Geometry: final body of the model. Coordinates: model frame, mm. Face numbers are marked on the shaded views. A direction names the side the tool comes from. Round coordinates to 2 decimals unless told otherwise and drop trailing zeros. Write each loop counter-clockwise with the first axis right and the second up, starting at its lowest first coordinate (ties: lowest second). Pieces come first, ordered by that corner, then holes. Notation, with made-up numbers: (40.5, 86.5) -> (75.5, 86.5) arc R15 cw to (75.5, 104.5) -> close; hole circle Ø3 at (80.5, -16.5). An arc over 180 degrees is marked (long way). One line per item, written item: value. Start each with the question number.
from build123d import *

# Parameters (mm, degrees)
CROQUIS3_R                 = 12
SALIENTE_EXTRUIR1_DEPTH    = 4
CROQUIS4_R                 = 3.95
SALIENTE_EXTRUIR2_DEPTH    = 35
CORTAR_EXTRUIR1_START      = -20
CORTAR_EXTRUIR1_DEPTH      = 20
CROQUIS7_R                 = 12
CORTAR_EXTRUIR2_DEPTH      = 2
CORTAR_EXTRUIR3_DEPTH      = 41.706264874
CORTAR_EXTRUIR3_DEPTH_BACK = 41.706264874
CROQUIS8_R                 = 0.726366889


with BuildPart() as part:
    # Croquis3 → Saliente-Extruir1 (new body)
    with BuildSketch(Plane(origin=(0, 0, 0), x_dir=(1, 0, 0), z_dir=(0, 1, 0))):
        with Locations(Location((0, 0, 0), (0, 0, 270))):
            Circle(CROQUIS3_R)
    extrude(amount=SALIENTE_EXTRUIR1_DEPTH)

    # Croquis4 → Saliente-Extruir2 (add)
    with BuildSketch(Plane(origin=(0, 4, 0), x_dir=(1, 0, 0), z_dir=(0, 1, 0))):
        with Locations(Location((0, 0, 0), (0, 0, 270))):
            Circle(CROQUIS4_R)
    extrude(amount=SALIENTE_EXTRUIR2_DEPTH)

    # Croquis5 → Cortar-Extruir1 (cut)
    with BuildSketch(Plane(origin=(0, 39, 0), x_dir=(1, 0, 0), z_dir=(0, 1, 0)).offset(CORTAR_EXTRUIR1_START)):
        with BuildLine():
            Line((2.626785107, 2.95), (-2.626785107, 2.95))
            ThreePointArc((-2.626785107, 2.95), (0, 3.95), (2.626785107, 2.95))
        make_face()
    extrude(amount=CORTAR_EXTRUIR1_DEPTH, mode=Mode.SUBTRACT)

    # Croquis7 → Cortar-Extruir2 (cut)
    with BuildSketch(Plane.XZ):
        with Locations(Location((0, 0, 0), (0, 0, 270))):
            Circle(CROQUIS7_R)
    extrude(amount=-CORTAR_EXTRUIR2_DEPTH, mode=Mode.SUBTRACT)

    # Croquis8 → Cortar-Extruir3 (cut, two sides: drawn at the far end of the back side and taken through both)
    with BuildSketch(Plane.XZ.offset(-2).offset(-CORTAR_EXTRUIR3_DEPTH_BACK)):
        with Locations(Location((0, 8, 0), (0, 0, 270))):
            Circle(CROQUIS8_R)
        with Locations(Location((0, -8, 0), (0, 0, 270))):
            Circle(CROQUIS8_R)
    extrude(amount=CORTAR_EXTRUIR3_DEPTH + CORTAR_EXTRUIR3_DEPTH_BACK, mode=Mode.SUBTRACT)


solid = part.part
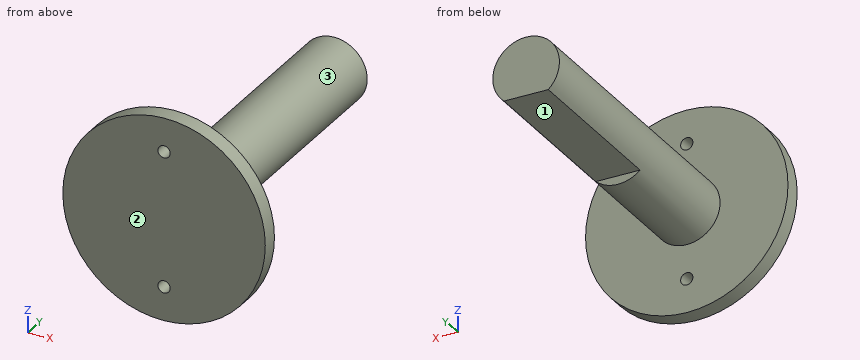
(1) Section query D-D (y = 21.5). Output: boundary loops of the cut face in (x, z), and give its area (3 significant figures).
(2) Pin query (flat end, axial travel): pin 1 (3 mm diameter, centred on x = -2.5, y = 26.5, fed in from -Z); pin 2 (12 mm diameter, centred on x = 6, z = 0.5, fed in from +Y); pin 3 (1 mm diameter, centred on x = 4, y = 15.5, fed in from +Z); pin 4 (12 mm diameter, centred on x = 0.5, y = 27.5, fed in from +Z). Return the tip coordinate at first contact, or that it passes through.
(3) Section query A-A (x = 0). Output: boundary loops of the cut face in (y, z).
(4) Set-up query: the marked faces 1, 2 and 3. Return all of +Z, -Z, +X, -X, +Y, -Y with unobstructed straight access to the full face (end or side cutting, diameter ignored); none if empty.
(5) Section query B-B (z = 8). Output: boundary loops of the cut face in (x, y), and give its area (3 significant figures).
(6) Line query: probe 1 along Y at (x, z) = (-6.5, -4); probe 2 along X at (y, z) = (2.9, 8); probe 3 along X at (y, z) = (18.5, -1.5). Output: solid intervals per line, ascending.
(7) Section query C-C (z = 0). Output: boundary loops of the cut face in (x, y).
Results list:
1. outline: (-2.63, -2.95) -> (2.63, -2.95) arc R3.95 ccw (long way) to start
1. area: 45.4 mm^2
2. pin 1: stops at z = -2.95
2. pin 2: stops at y = 39
2. pin 3: stops at z = 1.83
2. pin 4: stops at z = 3.95
3. outline: (2, -12) -> (4, -12) -> (4, -8.73) -> (2, -8.73) -> close; (2, -7.27) -> (4, -7.27) -> (4, -3.95) -> (19, -3.95) -> (19, -2.95) -> (39, -2.95) -> (39, 3.95) -> (4, 3.95) -> (4, 7.27) -> (2, 7.27) -> close; (2, 8.73) -> (4, 8.73) -> (4, 12) -> (2, 12) -> close
4. face 1: -Z, +X, -X, +Y
4. face 2: +Z, -Z, +X, -X, -Y
4. face 3: +Y
5. outline: (-8.94, 2) -> (-0.73, 2) -> (-0.73, 4) -> (-8.94, 4) -> close; (0.73, 2) -> (8.94, 2) -> (8.94, 4) -> (0.73, 4) -> close
5. area: 32.9 mm^2
6. probe 1: y = 2 to 4
6. probe 2: x = -8.94 to -0.73, 0.73 to 8.94
6. probe 3: x = -3.65 to 3.65
7. outline: (-12, 2) -> (12, 2) -> (12, 4) -> (3.95, 4) -> (3.95, 39) -> (-3.95, 39) -> (-3.95, 4) -> (-12, 4) -> close
